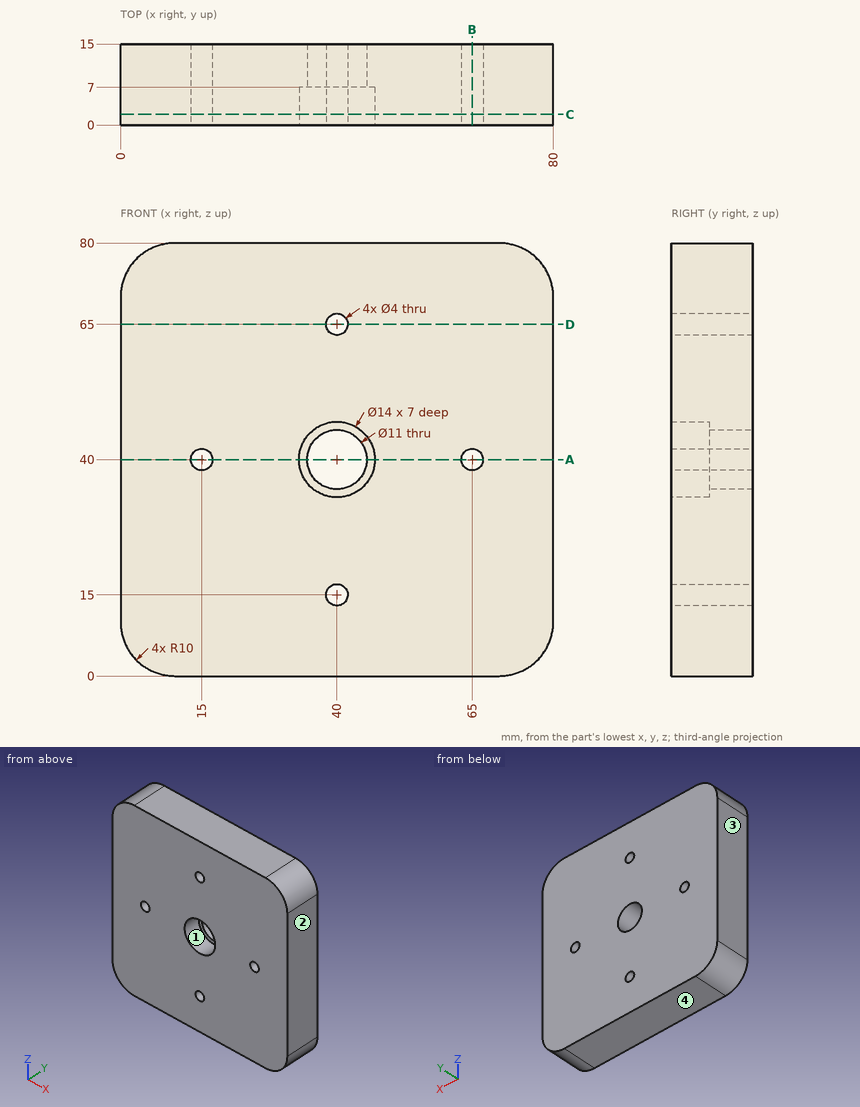
Study the drawing (mm; zero at the part's minimum x, y, z) and answer. Coordinates: 2 decimals unless noted, no trailing zeros. Order: outer loops, then holes, each group sorted by start corner. A loop starts at its lowest first (then second) coordinate and runs counter-clockwise, first axis right, second up. Notation, with made-up numbers: M 3.5,33 L 46.5,33 A19 cw 46.5,65 Z; hole C -10,79.25 d9. An arc over 180 degrees is marked long. Answer as a JSON object with one key per item and string values. Group by question number.
1. Section C-C on y = 2 is taken. Write down the section's boundary in (x, z), then the cut area to 3 significant figures.
2. Determine the mould class of the marked faces 1, 2, 3 and 4 for opening direction X: released by +X, released by -X, zero draft, split by the parting line, or undercut.
3. Section D-D on z = 65 is taken. Write down the section's boundary in (x, y), then the cut area to 3 significant figures.
4. Straight lines are drawn through the part: line 1 (X direction, y = 3.75, z = 40); line 2 (X direction, y = 4.5, z = 65). For each, find the intervals that lie inside material, in ascending order.
5. Section B-B on x = 65 is taken. Write down the section's boundary in (y, z).
6. Section A-A on z = 40 is taken. Write down the section's boundary in (x, y), then the cut area to 3 significant figures.
Values follow:
{
 "1": {"outline": "M 0,10 A10 ccw 10,0 L 70,0 A10 ccw 80,10 L 80,70 A10 ccw 70,80 L 10,80 A10 ccw 0,70 Z; hole C 15,40 d4; hole C 40,40 d14; hole C 40,15 d4; hole C 40,65 d4; hole C 65,40 d4", "area": "6,110 mm2"},
 "2": {"face 1": "undercut", "face 2": "released by +X", "face 3": "released by -X", "face 4": "zero draft"},
 "3": {"outline": "M 0,0 L 38,0 L 38,15 L 0,15 Z; M 42,0 L 80,0 L 80,15 L 42,15 Z", "area": "1,140 mm2"},
 "4": {"line 1": "0 to 13, 17 to 33, 47 to 63, 67 to 80", "line 2": "0 to 38, 42 to 80"},
 "5": {"outline": "M 0,0 L 15,0 L 15,38 L 0,38 Z; M 0,42 L 15,42 L 15,80 L 0,80 Z"},
 "6": {"outline": "M 0,0 L 13,0 L 13,15 L 0,15 Z; M 17,0 L 33,0 L 33,7 L 34.5,7 L 34.5,15 L 17,15 Z; M 45.5,7 L 47,7 L 47,0 L 63,0 L 63,15 L 45.5,15 Z; M 67,0 L 80,0 L 80,15 L 67,15 Z", "area": "894 mm2"}
}
